from build123d import *

# Parameters (mm, degrees)
F0_W     = 75.7237523794
F0_H     = 55.7212531567
F1_DEPTH = 25.4
F1_TAPER = -3
F2_T     = -2.54
F3_R     = 5.08
F4_DEPTH = 2.5410001


# Not quite as in the source:
# - a feature of the source that left no trace in its solid (it failed there, or was rolled back) is left out


with BuildPart() as f1:
    # F0 (on Front) → F1 (new body)
    with BuildSketch(Plane.XZ):
        Rectangle(F0_W, F0_H)
    extrude(amount=-F1_DEPTH, taper=F1_TAPER)

    # F2
    f2_openings = [f1.faces().sort_by_distance(p)[0] for p in [
        (0, 25.4, 0),
    ]]
    offset(amount=F2_T, openings=f2_openings)

    # F3 (on face) → F4 (cut, through all)
    with BuildSketch(Plane(origin=(0, 2.54, 0), x_dir=(-1, 0, 0), z_dir=(0, 1, 0))):
        with Locations((12.7, 8.0962497741)):
            Circle(F3_R)
        with Locations((-12.7, 8.0962497741)):
            Circle(F3_R)
    extrude(amount=-F4_DEPTH, mode=Mode.SUBTRACT)


solid = f1.part
Part model, mm, in its own coordinate system. A direction names the side the tool comes from. Coordinates: 2 decimals unless noted, no trailing zeros. Return JSON: item names as keys, results as strings.
1. Flat gauge pins, fed straight in: pin 1 Ø1 at (x, z) = (25.5, -11.5) entering from +Y; pin 2 Ø9 at (x, z) = (-12.7, 8.1) entering from -Y; pin 3 Ø1 at (x, y) = (-12, 22.5) entering from -Z; pin 4 Ø8 at (x, y) = (0.5, 18.5) entering from -Z. Where does each tip first touch, or does it go through?
Determined:
{"pin 1": "y = 2.54", "pin 2": "through", "pin 3": "z = -29.07", "pin 4": "z = -29.04"}
2. Saw through at A-A, the plane y = 1.5. Count the separate pieces of the cut face and the enclosed holes in it, then the cut area to 3 significant figures.
Determined:
{"separate pieces": "1", "enclosed holes": "2", "area": "4,080 mm²"}
3. Probe L1, parallel to Y at x = -4.5, z = 6; L2, parallel to Z at x = 12.7, y = 1.2; L3, parallel to Z at x = 30, y = 10.25. List the from-to ranges inside material, lowest first.
Determined:
{"L1": "0 to 2.54", "L2": "-27.92 to 3.02, 13.18 to 27.92", "L3": "-28.4 to -25.85, 25.85 to 28.4"}
4. Pull direction X, two halves, no side cores. Call faces 1 (the face through (-1, 0, 0)), 2 (the face through (-36.06, 14.13, 0.37)), 3 (the face through (-0.513, 14.13, -26.058)): pulls with the +X half, pulls with the -X half, needs draft (parallel to the pull), parting line crosses it, or undercut.
Determined:
{"face 1": "needs draft", "face 2": "undercut", "face 3": "undercut"}
5. 3-axis set-ups, long thin cutter, end or side, ignore diameter. For faces 4 (the face through (36.06, 14.13, -0.37)), 5 (the face through (-2, 25.4, -27)): which of +Z, -Z, +X, -X, +Y, -Y reach the whole face in a straight line?
Determined:
{"face 4": "+Y", "face 5": "+Z, -Z, +X, -X, +Y"}
